```python
from build123d import *

# Parameters (mm, degrees)
SKETCH1_R           = 1.5
BOSS_EXTRUDE1_DEPTH = 15
SKETCH2_R           = 2.5
BOSS_EXTRUDE2_DEPTH = 2
CUT_EXTRUDE2_DEPTH  = 1.6


with BuildPart() as part:
    # Sketch1 → Boss-Extrude1 (new body)
    with BuildSketch(Plane(origin=(0, 0, 0), x_dir=(1, 0, 0), z_dir=(0, 1, 0))):
        Circle(SKETCH1_R)
    extrude(amount=BOSS_EXTRUDE1_DEPTH)

    # Sketch2 → Boss-Extrude2 (add)
    with BuildSketch(Plane(origin=(0, 15, 0), x_dir=(1, 0, 0), z_dir=(0, 1, 0))):
        Circle(SKETCH2_R)
    extrude(amount=BOSS_EXTRUDE2_DEPTH)

    # Sketch3 → Cut-Extrude2 (cut)
    with BuildSketch(Plane(origin=(0, 17, 0), x_dir=(1, 0, 0), z_dir=(0, 1, 0))):
        Polygon((0.997116077, -1.781560543), (2.041434727, -0.027252418), (1.04431865, 1.754308125), (-0.997116077, 1.781560543), (-2.041434727, 0.027252418), (-1.04431865, -1.754308125), align=None)
    extrude(amount=-CUT_EXTRUDE2_DEPTH, mode=Mode.SUBTRACT)


solid = part.part
```
Work out the finished part from the listing and answer in its coordinate system (mm). A direction names the side the tool comes from. Round coordinates to 2 decimals unless told otherwise and drop trailing zeros. Order: outer loops, then holes, each group sorted by start corner. A loop starts at its lowest first (then second) coordinate and runs counter-clockwise, first axis right, second up.
Q1. A cutting plane is placed at B-B, the plane y = 10.5. Determine the outline of the cut face in (x, z), then the cut area to 3 significant figures.
Solution:
outline: circle Ø3 at (0, 0)
area: 7.07 mm2
Q2. A cutting plane is placed at C-C, the plane z = 0.4. Determine the outline of the cut face in (x, y).
Solution:
outline: (-2.47, 15) - (-1.45, 15) - (-1.45, 0) - (1.45, 0) - (1.45, 15) - (2.47, 15) - (2.47, 17) - (1.82, 17) - (1.82, 15.4) - (-1.8, 15.4) - (-1.8, 17) - (-2.47, 17) - close
Q3. Find the intervals of material crossed by line 1 along Y through (x, z) = (-0.15, 1.05); line 2 along Y through (x, z) = (-0.55, 1.8); line 3 along Z through (x, y) = (-1.9, 16.25), in increasing order.
Solution:
line 1: y = 0 to 15.4
line 2: y = 15 to 17
line 3: z = -1.62 to -0.26, 0.23 to 1.62
Q4. A cutting plane is placed at A-A, the plane x = -0.3. Determine the outline of the cut face in (y, z), then the cut area to 3 significant figures.
Solution:
outline: (0, -1.47) - (15, -1.47) - (15, -2.48) - (17, -2.48) - (17, -1.77) - (15.4, -1.77) - (15.4, 1.76) - (17, 1.76) - (17, 2.48) - (15, 2.48) - (15, 1.47) - (0, 1.47) - close
area: 48.4 mm2
Q5. Given pin 1 Ø1 at (x, y) = (-2, 15) entering from -Z; pin 2 Ø1 at (y, z) = (6.5, 0.5) entering from -X; pin 3 Ø3 at (y, z) = (9.5, 0) entering from +X, each flat-ended and moving along its own axis, determine where each tip first touches the part or whether it passes through.
Solution:
pin 1: stops at z = -2
pin 2: stops at x = -1.5
pin 3: stops at x = 1.5
Q6. The mould has two halves that part along Z. Classify faces 1 (the flat face through (0, 0, 0)), 2 (the cylindrical face through (-1.5, 7.4, -0.07)), 3 (the flat face through (1.51, 16.21, 0.92)): pulls with the +Z half, pulls with the -Z half, needs draft (parallel to the pull), parting line crosses it, or undercut.
Solution:
face 1: needs draft
face 2: parting line crosses it
face 3: undercut
Q7. A tool of negligible diameter and unlimited length cuts with its end or side. For faces 4 (the flat face through (0, 15.4, 0)), 5 (the flat face through (0, 15, 2)), 6 (the cylindrical face through (-0.54, 15.99, 2.44)), from which of +Z, -Z, +X, -X, +Y, -Y can it reach the whole face along a straight path? Write none if from no direction.
Solution:
face 4: +Y
face 5: -Y
face 6: +Y, -Y
